For this review, take the finished solid that the model builds, in its own axes (mm). A direction names the side the tool comes from. Round coordinates to 2 decimals unless told otherwise and drop trailing zeros. Order: outer loops, then holes, each group sorted by start corner. A loop starts at its lowest first (then second) coordinate and runs counter-clockwise, first axis right, second up. Notation, with made-up numbers: M 32,-6 L 53,-6 A33 ccw 53,24 Z; hole C -36.5,66 d11. An arc over 180 degrees is marked long. Put each result on its own line as item: value.
from build123d import *

# Parameters (mm, degrees)
SKETCH_1_R               = 24.5
EXTRUDE_1_DEPTH          = 39
SKETCH_2_R               = 20
CUT_EXTRUDE_1_DEPTH      = 36
SKETCH_3_R               = 15
CUT_EXTRUDE_2_DEPTH      = 50.964987741
CUT_EXTRUDE_START        = 33
SKETCH_4_R               = 21.75
CUT_EXTRUDE_3_DEPTH      = 1.5
EXTRUDE_START            = -21
SKETCH_5_R               = 41
SKETCH_5_R_2             = 24.5
EXTRUDE_2_DEPTH          = 5
SKETCH_6_R               = 4.25
CUT_EXTRUDE_4_DEPTH      = 63.377880695
PATTERN_CIRCULAR_1_COUNT = 4


with BuildPart() as part:
    # 草图1 → 凸台-拉伸1 (new body)
    with BuildSketch(Plane.XY):
        Circle(SKETCH_1_R)
    extrude(amount=EXTRUDE_1_DEPTH)

    # 草图2 → 切除-拉伸1 (cut)
    with BuildSketch(Plane.XY.offset(39)):
        Circle(SKETCH_2_R)
    extrude(amount=-CUT_EXTRUDE_1_DEPTH, mode=Mode.SUBTRACT)

    # 草图3 → 切除-拉伸2 (cut, through all)
    with BuildSketch(Plane.XY.offset(3)):
        Circle(SKETCH_3_R)
    extrude(amount=-CUT_EXTRUDE_2_DEPTH, mode=Mode.SUBTRACT)

    # 草图4 → 切除-拉伸3 (cut)
    with BuildSketch(Plane.XY.offset(3).offset(CUT_EXTRUDE_START)):
        Circle(SKETCH_4_R)
    extrude(amount=CUT_EXTRUDE_3_DEPTH, mode=Mode.SUBTRACT)

    # 草图5 → 凸台-拉伸2 (add)
    with BuildSketch(Plane.XY.offset(39).offset(EXTRUDE_START)):
        Circle(SKETCH_5_R)
        Circle(SKETCH_5_R_2, mode=Mode.SUBTRACT)
    extrude(amount=EXTRUDE_2_DEPTH)

    # 草图6 → 切除-拉伸4 (cut, through all)
    with BuildSketch(Plane.XY.offset(23)):
        with Locations((32.5, 0)):
            Circle(SKETCH_6_R)
    cut_extrude_4 = extrude(amount=-CUT_EXTRUDE_4_DEPTH, mode=Mode.SUBTRACT)

    # 阵列(圆周)1: 切除-拉伸4 ×4 about axis
    pattern_circular_1_axis = Axis((0, 0, 0), (0, 0, 1))
    for i in range(1, PATTERN_CIRCULAR_1_COUNT):
        add(cut_extrude_4.rotate(pattern_circular_1_axis, i * 360 / PATTERN_CIRCULAR_1_COUNT), mode=Mode.SUBTRACT)


solid = part.part
(1) Add section D-D on y = 0. State how many separate pieces and enclosed holes the cut face has, then the cut area to 3 significant figures.
A:
separate pieces: 4
enclosed holes: 0
area: 456 mm2
(2) For faces 1 (the face through (-14.985, 0.66, 1.521)), 2 (the face through (18, -18, 18)), 3 (the face through (10, -18, 37.5)), 4 (the face through (18, -18, 23)), list the 3-axis set-ups (+Z, -Z, +X, -X, +Y, -Y) from which the entire face can be reached by the end or side of a thin tool; tool diameter is ignored.
A:
face 1: +Z, -Z
face 2: -Z
face 3: none
face 4: +Z
(3) Add section A-A on y = 32.5. Give the boundary of the cut face in (x, z) (3 decimals), then the cut area to 3 significant figures.
A:
outline: M -24.995,18 L -4.25,18 L -4.25,23 L -24.995,23 Z; M 4.25,18 L 24.995,18 L 24.995,23 L 4.25,23 Z
area: 207 mm2
(4) Draft analysis for pull direction Y (two halves, no side actions). For faces 5 (the face through (-9.2, -18, 39)), 6 (the face through (-9, -40, 20)), 7 (the face through (-4.336, -19.524, 19.731)), state which applies: released by +Y, released by -Y, zero draft, split by the parting line, or undercut.
A:
face 5: zero draft
face 6: split by the parting line
face 7: undercut
(5) To check wall thickness, follow L1, parallel to Y at x = 0, z = 16; L2, parallel to Z at x = -14.5, y = -23; L3, parallel to Y at x = -17, z = 36.5. State the ranges of each line that lie inside material, in increasing order.
A:
L1: y = -24.5 to -20, 20 to 24.5
L2: z = 18 to 23
L3: y = -17.64 to -13.57, 13.57 to 17.64
(6) Add section B-B on z = 21. Give the boundary of the cut face in (x, y).
A:
outline: C 0,0 d82; hole C -32.5,0 d8.5; hole C 0,0 d40; hole C 0,-32.5 d8.5; hole C 0,32.5 d8.5; hole C 32.5,0 d8.5
(7) Insertion check: pin 1 Ø10 at (y, z) = (17.5, 10.5) entering from +X; pin 2 Ø2 at (y, z) = (17.5, 24.5) entering from +X; pin 3 Ø13.5 at (x, y) = (0, -32.5) entering from -Z; pin 4 Ø1.5 at (y, z) = (32.5, 24.5) entering from -X. Each pin has a flat end and moves straight along its axis. Give the tip position at first contact, or say it passes through.
A:
pin 1: stops at x = 21.07
pin 2: stops at x = 18.11
pin 3: stops at z = 18
pin 4: passes through
